Check sheet for the modelled part. Datum: model origin and axes. Units: mm. Face numbers are marked on the shaded views. Round coordinates to 2 decimals unless told otherwise and drop trailing zeros. Loops run counter-clockwise (first coordinate to the right, second up) from the corner with the lowest first, then second, coordinate; pieces in that order, holes last. Notation, with made-up numbers: (6, 69) - (61, 69) arc R22 ccw to (61, 92) - close; hole circle Ø3 at (-5.5, 48.5). An arc over 180 degrees is marked (long way). Put each result on its own line as item: value.
```python
from build123d import *


with BuildPart() as part:
    # Sketch1 → Revolve1 (revolve)
    with BuildSketch(Plane.XY):
        with BuildLine():
            Line((2.983876441, 24), (2.983876441, 21))
            Line((2.983876441, 21), (3.983876441, 20))
            Line((3.983876441, 20), (14.983876441, 20))
            Line((14.983876441, 20), (14.983876441, 29.495))
            Line((14.983876441, 29.495), (9.023876441, 29.495))
            Line((9.023876441, 29.495), (4.783876441, 30.014855378))
            Line((4.783876441, 30.014855378), (3.783876441, 29))
            Line((3.783876441, 29), (3.783876441, 26.245704095))
            Line((3.783876441, 26.245704095), (7.463876441, 25.794508861))
            ThreePointArc((7.463876441, 25.794508861), (8.361130872, 24.89725443), (7.463876441, 24))
            Line((7.463876441, 24), (2.983876441, 24))
        make_face()
    revolve(axis=Axis((0, 0, 0), (1, 0, 0)))


solid = part.part
```
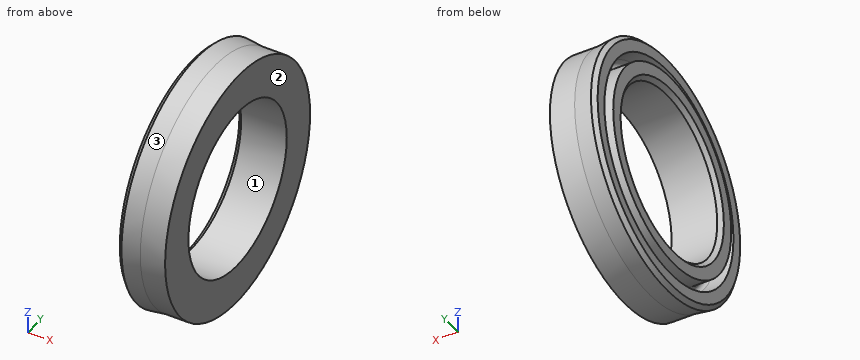
Item 1: Section check A-A on z = 0. Enter the section's corners in (x, y) (1 decimal), then the cut area to 3 significant figures.
Filled sheet:
outline: (3, -24) - (7.5, -24) arc R0.9 cw to (7.5, -25.8) - (3.8, -26.2) - (3.8, -29) - (4.8, -30) - (9, -29.5) - (15, -29.5) - (15, -20) - (4, -20) - (3, -21) - close; (3, 21) - (4, 20) - (15, 20) - (15, 29.5) - (9, 29.5) - (4.8, 30) - (3.8, 29) - (3.8, 26.2) - (7.5, 25.8) arc R0.9 cw to (7.5, 24) - (3, 24) - close
area: 203 mm²
Item 2: Section check C-C on x = 12. Enter the section's corners in (y, z) (3 decimals).
Filled sheet:
outline: circle Ø58.99 at (0, 0); hole circle Ø40 at (0, 0)
Item 3: Go/stop test with flat-tipped pins: pin 1 (4 mm diameter, centred on x = 6.5, y = 23, fed in from -Z); pin 2 (1 mm diameter, centred on x = 12, y = -20.5, fed in from +Z); pin 3 (1.5 mm diameter, centred on x = 13, z = -22, fed in from +Y). Record where each tip stops, or that it passes through.
Filled sheet:
pin 1: z = -21.18
pin 2: z = 21.68
pin 3: y = 20.45
Item 4: Release check for a two-part mould opening along Z. For the marked faces 1, 2 and 3 record: +Z half, -Z half, draft (parallel to the pull), parting line (faces both ways), or undercut.
Filled sheet:
face 1: undercut
face 2: draft
face 3: parting line
Item 5: Thickness scan on line 1 (Z direction, x = 6, y = -15) (3 decimals); line 2 (Y direction, x = 4.25, z = 10); line 3 (Y direction, x = 7.25, z = -15) (3 decimals). Record the ranges inside material, lowest first. Write a range as from..to.
Filled sheet:
line 1: -25.826..-21.205, -18.735..-13.229, 13.229..18.735, 21.205..25.826
line 2: -27.72..-24.2, -21.82..-17.32, 17.32..21.82, 24.2..27.72
line 3: -25.648..-21.017, -18.735..-13.229, 13.229..18.735, 21.017..25.648
